Geometry: final body of the model. Coordinates: model frame, mm. Give positions to 0.01 mm unless a question says otherwise; leave off trailing zeros. Order: outer loops, then holes, each group sorted by start corner. A loop starts at its lowest first (then second) coordinate and runs counter-clockwise, first axis right, second up. Notation, with made-up numbers: (60.25, 40) - (105.25, 40) arc R28 cw to (105.25, 63) - close; hole circle Ø7 at (-11.75, 16.25). An arc over 180 degrees is marked (long way). Write item = value, one per line. Start each with the question number.
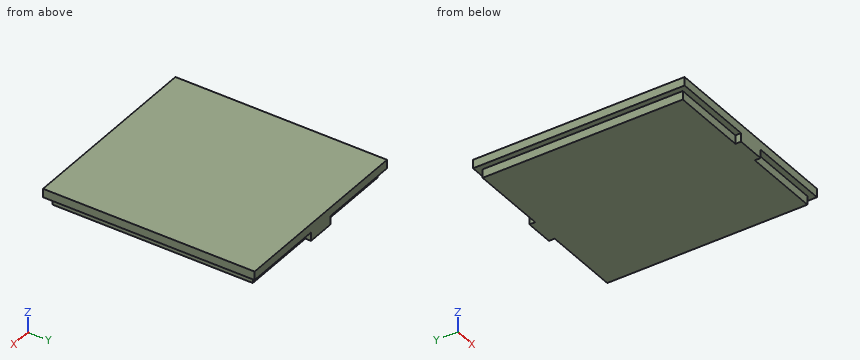
from build123d import *

# Parameters (mm, degrees)
SKETCH_W        = 34
SKETCH_H        = 37
PAD_DEPTH       = 15
SKETCH001_W     = 32
SKETCH001_H     = 35
POCKET_DEPTH    = 1.5
SKETCH002_W     = 30
SKETCH002_H     = 33
POCKET001_DEPTH = 10
SKETCH003_W     = 5
SKETCH003_H     = 5
POCKET002_DEPTH = 300
SKETCH004_W     = 34
SKETCH004_H     = 37
PAD001_DEPTH    = 1.5


with BuildPart() as pocket002:
    # Sketch → Pad (new body)
    with BuildSketch(Plane.XY):
        Rectangle(SKETCH_W, SKETCH_H)
    extrude(amount=PAD_DEPTH)

    # Sketch001 → Pocket (cut)
    with BuildSketch(Plane.XY.offset(15)):
        Rectangle(SKETCH001_W, SKETCH001_H)
    extrude(amount=-POCKET_DEPTH, mode=Mode.SUBTRACT)

    # Sketch002 → Pocket001 (cut)
    with BuildSketch(Plane.XY.offset(13.5)):
        Rectangle(SKETCH002_W, SKETCH002_H)
    extrude(amount=-POCKET001_DEPTH, mode=Mode.SUBTRACT)

    # Sketch003 → Pocket002 (cut)
    with BuildSketch(Plane.XZ.offset(18.5)):
        with Locations((0, 12.5)):
            Rectangle(SKETCH003_W, SKETCH003_H)
    extrude(amount=-POCKET002_DEPTH, mode=Mode.SUBTRACT)


with BuildPart() as cut:
    # Pad001 base: copy of Pocket002
    add(pocket002.part)

    # Sketch004 → Pad001 (new body, symmetric)
    with BuildSketch(Plane.XY.offset(15)):
        Rectangle(SKETCH004_W, SKETCH004_H)
    extrude(amount=PAD001_DEPTH, both=True)

    # Cut: cut Pocket002
    add(pocket002.part, mode=Mode.SUBTRACT)


solid = cut.part
Q1. Section A-A, the plane z = 14.3. Return the cut outline in (x, y), then the cut area to 3 significant figures.
Q2. Section B-B, the plane y = -15. Return the cut outline in (x, z).
Q3. Section C-C, the plane x = 11. Return the cut outline in (y, z), then the cut area to 3 significant figures.
Q4. Material intervals for line 1 along X through (y, z) = (-13, 14.5); line 2 along Y through (x, z) = (-7, 14.4), sorted ascending. Write a range as from..to.
Q5. Contact query for flat-ended pins moving along their axis: pin 1 (0.8 mm diameter, centred on y = -4, z = 14.5, fed in from -X); pin 2 (0.8 mm diameter, centred on y = -18, z = 14, fed in from -X); pin 3 (1.2 mm diameter, centred on x = -10, z = 14, fed in from +Y). Output: stop coordinate, or through.
The answers:
q1.outline = (-16, -17.5) - (-2.5, -17.5) - (-2.5, -18.5) - (2.5, -18.5) - (2.5, -17.5) - (16, -17.5) - (16, 17.5) - (2.5, 17.5) - (2.5, 18.5) - (-2.5, 18.5) - (-2.5, 17.5) - (-16, 17.5) - close
q1.area = 1,130 mm²
q2.outline = (-17, 15) - (-16, 15) - (-16, 13.5) - (16, 13.5) - (16, 15) - (17, 15) - (17, 16.5) - (-17, 16.5) - close
q3.outline = (-18.5, 15) - (-17.5, 15) - (-17.5, 13.5) - (17.5, 13.5) - (17.5, 15) - (18.5, 15) - (18.5, 16.5) - (-18.5, 16.5) - close
q3.area = 108 mm²
q4.line_1 = -16..16
q4.line_2 = -17.5..17.5
q5.pin_1 = -16
q5.pin_2 = -2.5
q5.pin_3 = 17.5
